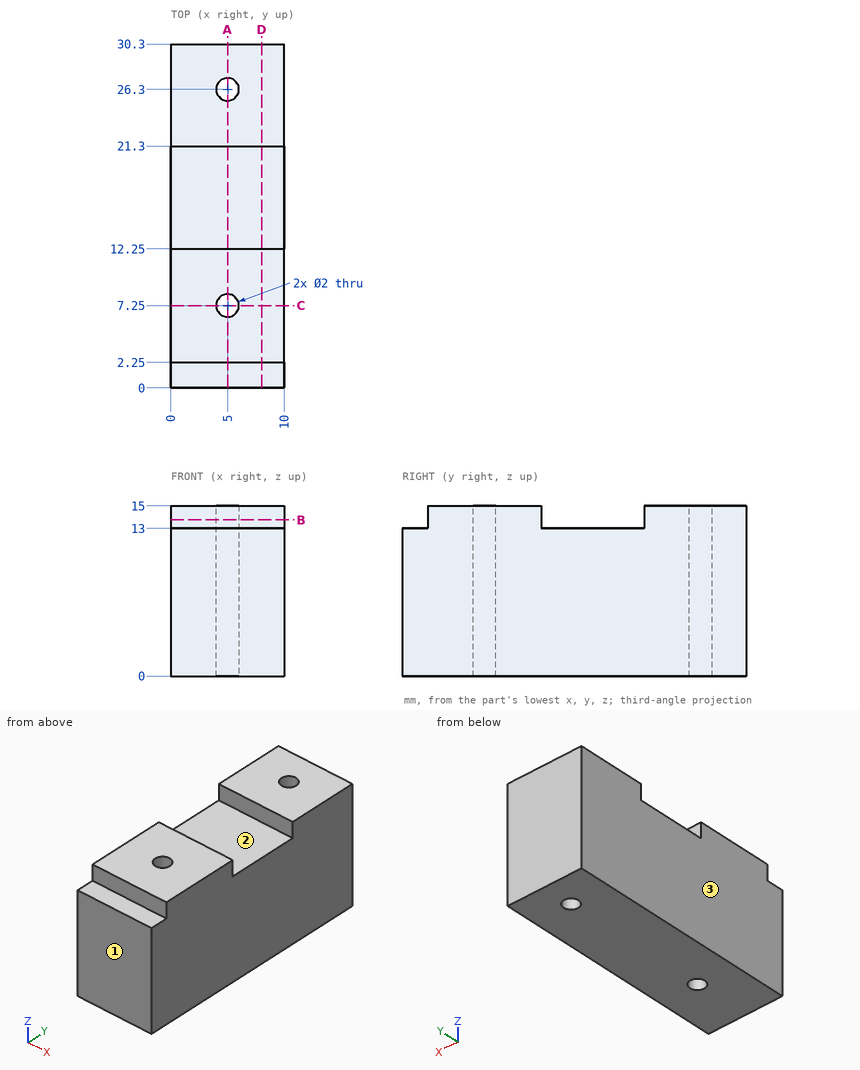
For this review, use the dimensioned drawing (mm, ordinates from the lowest corner) and the shaded views. Coordinates: 2 decimals unless noted, no trailing zeros. Loops run counter-clockwise (first coordinate to the right, second up) from the corner with the lowest first, then second, coordinate; pieces in that order, holes last. Notation, with made-up numbers: (64.5, 40) - (117.5, 40) arc R26 cw to (117.5, 64) - close; hole circle Ø5 at (43, 84.25). An arc over 180 degrees is marked (long way). Use CSV: the item, a comma, the result in double quotes. Start each with the question number.
1) Consider section D-D on x = 8. Write out the cut boundary in (y, z), then the cut area to 3 significant figures.
2) Consider section A-A on x = 5. Write out the cut boundary in (y, z).
3) Consider section B-B on z = 13.75. Write out the cut boundary in (x, y), then the cut area to 3 significant figures.
4) Wall thickness on L1, parallel to Y at x = 5, z = 10.5; L2, parallel to Y at x = 4.5, z = 2.5; L3, parallel to Z at x = 7.5, y = 19: over which ranges is each line inside the solid? List them lowest first. Write a range as from..to.
5) Consider section C-C on y = 7.25. Write out the cut boundary in (x, z).
6) For pin 1 Ø1.8 at (x, y) = (6.5, 0.5) entering from +Z, flat-tipped, find the tip position at first contact; note if it passes through.
7) The part is to be moulded in two halves that separate along Y. For the marked faces 1, 2 and 3, say which applies: +Y half, -Y half, draft (parallel to the pull), parting line (faces both ways), or undercut.
Geometry says:
1,outline,"(0, 0) - (30.3, 0) - (30.3, 15) - (21.3, 15) - (21.3, 13) - (12.25, 13) - (12.25, 15) - (2.25, 15) - (2.25, 13) - (0, 13) - close"
1,area,"432 mm^2"
2,outline,"(0, 0) - (6.25, 0) - (6.25, 15) - (2.25, 15) - (2.25, 13) - (0, 13) - close; (8.25, 0) - (25.3, 0) - (25.3, 15) - (21.3, 15) - (21.3, 13) - (12.25, 13) - (12.25, 15) - (8.25, 15) - close; (27.3, 0) - (30.3, 0) - (30.3, 15) - (27.3, 15) - close"
3,outline,"(0, 2.25) - (10, 2.25) - (10, 12.25) - (0, 12.25) - close; (0, 21.3) - (10, 21.3) - (10, 30.3) - (0, 30.3) - close; hole circle Ø2 at (5, 7.25); hole circle Ø2 at (5, 26.3)"
3,area,"184 mm^2"
4,L1,"0..6.25, 8.25..25.3, 27.3..30.3"
4,L2,"0..6.38, 8.12..25.43, 27.17..30.3"
4,L3,"0..13"
5,outline,"(0, 0) - (4, 0) - (4, 15) - (0, 15) - close; (6, 0) - (10, 0) - (10, 15) - (6, 15) - close"
6,pin 1,"z = 13"
7,face 1,"-Y half"
7,face 2,"undercut"
7,face 3,"draft"
